```python
from build123d import *

# Parameters (mm, degrees)
SKETCH2_W                             = 50
SKETCH2_H                             = 92.5
BASE_FLANGE1_DEPTH                    = 2
TAP_DRILL_FOR_M6_TAP1_AT_2_COUNT      = 2
TAP_DRILL_FOR_M6_TAP1_AT_2_PITCH      = 34.456169259
TAP_DRILL_FOR_M6_TAP1_AT_3_COUNT      = 2
TAP_DRILL_FOR_M6_TAP1_AT_3_PITCH      = 27.5
TAP_DRILL_FOR_M6_TAP1_AT_4_COUNT      = 2
TAP_DRILL_FOR_M6_TAP1_AT_4_PITCH      = 20.76
TAP_DRILL_FOR_M10X1_0_TAP1_AT_2_COUNT = 2
TAP_DRILL_FOR_M10X1_0_TAP1_AT_2_PITCH = 32.5
TAP_DRILL_FOR_M10X1_0_TAP1_AT_3_COUNT = 2
TAP_DRILL_FOR_M10X1_0_TAP1_AT_3_PITCH = 46.67440412
TAP_DRILL_FOR_M10X1_0_TAP1_AT_4_COUNT = 2
TAP_DRILL_FOR_M10X1_0_TAP1_AT_4_PITCH = 33.5


# Sheet-metal steps are written as plain solids
with BuildPart() as part:
    # Sketch2 → Base-Flange1 (new body)
    with BuildSketch(Plane(origin=(0, 0, 0), x_dir=(1, 0, 0), z_dir=(0, 1, 0))):
        with Locations((-2.5, -1.25)):
            Rectangle(SKETCH2_W, SKETCH2_H)
    extrude(amount=-BASE_FLANGE1_DEPTH)

    # Sketch8 → Tap Drill for M6 Tap1 (revolve, cut)
    with BuildSketch(Plane(origin=(11.25, 0, -11.74), x_dir=(0, 0, 1), z_dir=(1, 0, 0))):
        Polygon((0, 0), (0, 2), (2.5, 2), (2.5, 0.025), (2.525, 0), align=None)
    tap_drill_for_m6_tap1 = revolve(axis=Axis((11.25, 6.35, -11.74), (0, -1, 0)), mode=Mode.SUBTRACT)

    # Tap Drill for M6 Tap1 at 2: Tap Drill for M6 Tap1 ×2
    with Locations(*[Vector(-0.7981154200092394, 0, -0.6025045861597035) * (i * TAP_DRILL_FOR_M6_TAP1_AT_2_PITCH) for i in range(1, TAP_DRILL_FOR_M6_TAP1_AT_2_COUNT)]):
        add(tap_drill_for_m6_tap1, mode=Mode.SUBTRACT)

    # Tap Drill for M6 Tap1 at 3: Tap Drill for M6 Tap1 ×2
    with Locations(*[(-i * TAP_DRILL_FOR_M6_TAP1_AT_3_PITCH, 0, 0) for i in range(1, TAP_DRILL_FOR_M6_TAP1_AT_3_COUNT)]):
        add(tap_drill_for_m6_tap1, mode=Mode.SUBTRACT)

    # Tap Drill for M6 Tap1 at 4: Tap Drill for M6 Tap1 ×2
    with Locations(*[(0, 0, -i * TAP_DRILL_FOR_M6_TAP1_AT_4_PITCH) for i in range(1, TAP_DRILL_FOR_M6_TAP1_AT_4_COUNT)]):
        add(tap_drill_for_m6_tap1, mode=Mode.SUBTRACT)

    # Sketch15 → Tap Drill for M10x1.0 Tap1 (revolve, cut)
    with BuildSketch(Plane(origin=(-19.417070164, 0, 6.087287234), x_dir=(0, 0, 1), z_dir=(1, 0, 0))):
        Polygon((0, 0), (0, 2), (4.5, 2), (4.5, 0.025), (4.525, 0), align=None)
    tap_drill_for_m10x1_0_tap1 = revolve(axis=Axis((-19.417070164, 6.35, 6.087287234), (0, -1, 0)), mode=Mode.SUBTRACT)

    # Tap Drill for M10x1.0 Tap1 at 2: Tap Drill for M10x1.0 Tap1 ×2
    with Locations(*[(0, 0, i * TAP_DRILL_FOR_M10X1_0_TAP1_AT_2_PITCH) for i in range(1, TAP_DRILL_FOR_M10X1_0_TAP1_AT_2_COUNT)]):
        add(tap_drill_for_m10x1_0_tap1, mode=Mode.SUBTRACT)

    # Tap Drill for M10x1.0 Tap1 at 3: Tap Drill for M10x1.0 Tap1 ×2
    with Locations(*[Vector(0.7177381400208425, 0, 0.6963131209157426) * (i * TAP_DRILL_FOR_M10X1_0_TAP1_AT_3_PITCH) for i in range(1, TAP_DRILL_FOR_M10X1_0_TAP1_AT_3_COUNT)]):
        add(tap_drill_for_m10x1_0_tap1, mode=Mode.SUBTRACT)

    # Tap Drill for M10x1.0 Tap1 at 4: Tap Drill for M10x1.0 Tap1 ×2
    with Locations(*[(i * TAP_DRILL_FOR_M10X1_0_TAP1_AT_4_PITCH, 0, 0) for i in range(1, TAP_DRILL_FOR_M10X1_0_TAP1_AT_4_COUNT)]):
        add(tap_drill_for_m10x1_0_tap1, mode=Mode.SUBTRACT)

    # Sketch18 → Tap Drill for M36x2.0 Tap1 (revolve, cut)
    with BuildSketch(Plane(origin=(-2.667070164, 0, 22.337287234), x_dir=(0, 0, 1), z_dir=(1, 0, 0))):
        Polygon((0, 0), (0, 2), (17, 2), (17, 0.025), (17.025, 0), align=None)
    revolve(axis=Axis((-2.667070164, 6.35, 22.337287234), (0, -1, 0)), mode=Mode.SUBTRACT)


solid = part.part
```
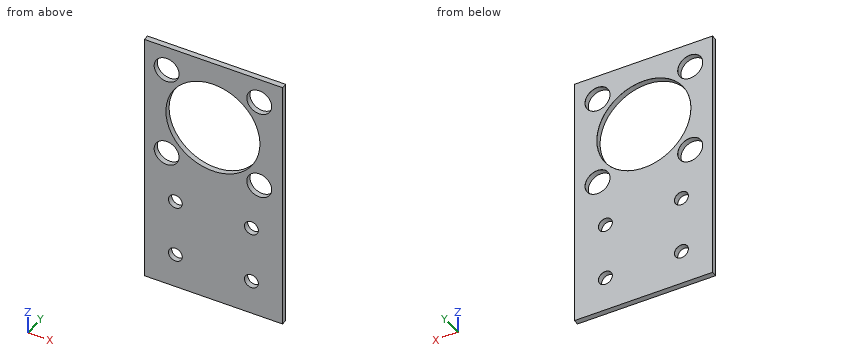
CAD build for the part. Positions are in the model's coordinates, mm. Coordinates: 2 decimals unless noted, no trailing zeros. Write each loop counter-clockwise with the first axis right and the second up, starting at its lowest first coordinate (ties: lowest second). Pieces come first, ordered by that corner, then holes.
(1) Flat gauge pins, fed straight in: pin 1 (5.5 mm diameter, centred on x = 14.08, z = 6.09, fed in from +Y); pin 2 (3 mm diameter, centred on x = 11, z = -33.5, fed in from -Y). Where does each tip first touch, or does it go through?
(2) Drill centre lines: probe 1 along X at (y, z) = (-0.8, -12); probe 2 along Z at (x, y) = (-16.25, -1.4); probe 3 along X at (y, z) = (-0.8, 23). Where is each one in solid material? Low to high.
(3) Cut at B-B, the plane y = -1.25. Count the separate pieces of the cut face and the enclosed holes in it, and give its area (3 significant figures).
(4) Cut at A-A, the plane z = -32.5. List the corners of the cut face in (x, y) (3 decimals).
Geometry says:
1. pin 1: passes through
1. pin 2: stops at y = -2
2. probe 1: x = -27.5 to -18.74, -13.76 to 8.76, 13.74 to 22.5
2. probe 2: z = -45 to -35, -30 to -14.24, -9.24 to 2.89, 9.28 to 12.11, 32.56 to 35.39, 41.78 to 47.5
2. probe 3: x = -27.5 to -19.65, 14.32 to 22.5
3. separate pieces: 1
3. enclosed holes: 9
3. area: 3,380 mm2
4. outline: (-27.5, -2) - (-18.75, -2) - (-18.75, -0.025) - (-18.775, 0) - (-27.5, 0) - close; (-13.75, -2) - (8.75, -2) - (8.75, -0.025) - (8.725, 0) - (-13.725, 0) - (-13.75, -0.025) - close; (13.75, -2) - (22.5, -2) - (22.5, 0) - (13.775, 0) - (13.75, -0.025) - close
